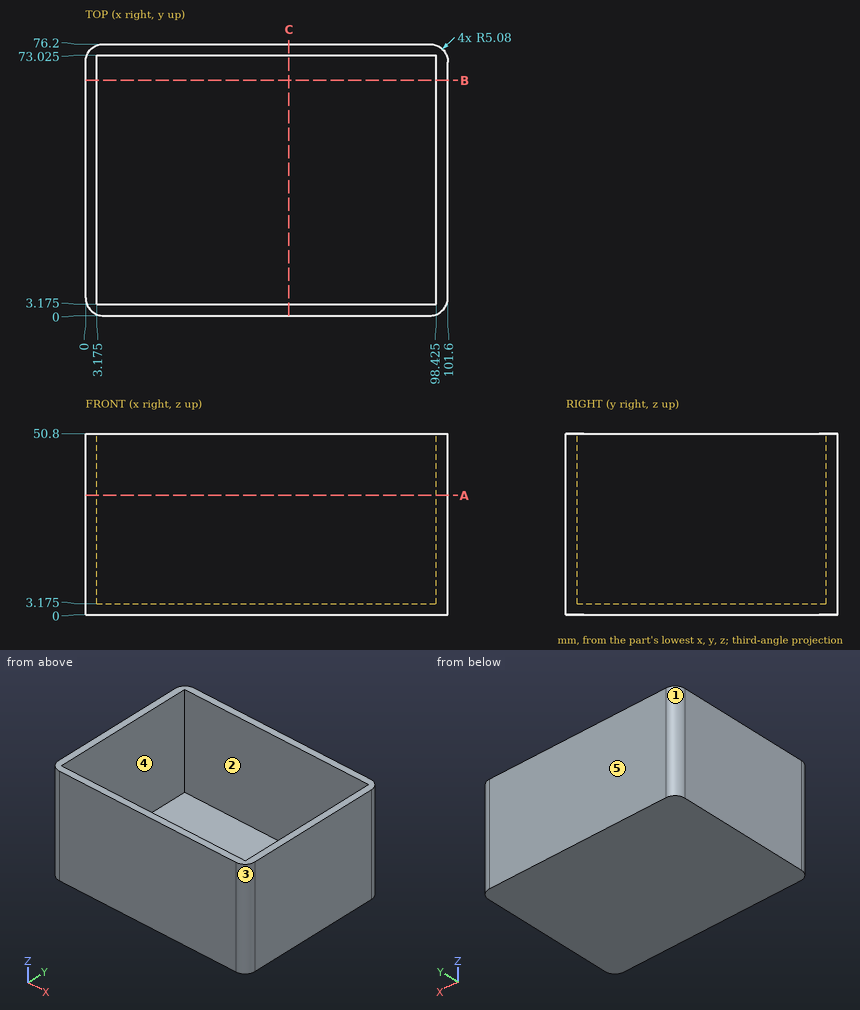
Verification items for this drawing (mm, ordinates from the low corner). A direction names the side the tool comes from. Coordinates: 2 decimals unless noted, no trailing zeros. Order: outer loops, then holes, each group sorted by start corner. A loop starts at its lowest first (then second) coordinate and runs counter-clockwise, first axis right, second up. Notation, with made-up numbers: M -7.75,11 L 18.25,11 A20 ccw 18.25,16 Z; hole C 37.25,26 d3. An arc over 180 degrees is marked long. One line per item, written item: value. Start each with the question number.
Item 1: Sectioned sample at C-C on x = 57. Record the cut outline in (y, z) (3 decimals), then the cut area to 3 significant figures.
Item 2: Access from +Z, -Z, +X, -X, +Y, -Y to the whole of each face (thin tool, end or side, straight path). Record for the marked faces 4 and 5.
Item 3: Sectioned sample at B-B on y = 66. Record the cut outline in (x, z) (3 decimals), then the cut area to 3 significant figures.
Item 4: Mould release check, pull along X, two halves, no side actions. Record for the marked faces 1, 2 and 3: pulls with the +X half, pulls with the -X half, needs draft (parallel to the pull), parting line crosses it, or undercut.
Item 5: Sectioned sample at A-A on z = 33.5. Record the cut outline in (x, y) (3 decimals).
Item 6: Depth check by flat-ended pin: P1, Ø24, axis at y = 54, z = 37.5, coming from the -X side; P2, Ø1.5, axis at x = 48.5, y = 33.5, coming from the +Z side (3 decimals). Enter the tip coordinate at first touch or a pass-through.
Item 7: Thickness scan on probe 1 along Y at (x, z) = (44.5, 18) (3 decimals); probe 2 along X at (y, z) = (54.5, 25.5) (3 decimals); probe 3 along Z at (x, y) = (24, 48) (3 decimals). Record the ranges inside material, lowest first.
Calculated:
1. outline: M 0,0 L 76.2,0 L 76.2,50.8 L 73.025,50.8 L 73.025,3.175 L 3.175,3.175 L 3.175,50.8 L 0,50.8 Z
1. area: 544 mm^2
2. face 4: +Z
2. face 5: +Z, -Z, +X, -X, +Y
3. outline: M 0,0 L 101.6,0 L 101.6,50.8 L 98.425,50.8 L 98.425,3.175 L 3.175,3.175 L 3.175,50.8 L 0,50.8 Z
3. area: 625 mm^2
4. face 1: pulls with the -X half
4. face 2: undercut
4. face 3: pulls with the +X half
5. outline: M 0,5.08 A5.08 ccw 5.08,0 L 96.52,0 A5.08 ccw 101.6,5.08 L 101.6,71.12 A5.08 ccw 96.52,76.2 L 5.08,76.2 A5.08 ccw 0,71.12 Z; hole M 3.175,3.175 L 98.425,3.175 L 98.425,73.025 L 3.175,73.025 Z
6. P1: x = 0
6. P2: z = 3.175
7. probe 1: 0 to 3.175, 73.025 to 76.2
7. probe 2: 0 to 3.175, 98.425 to 101.6
7. probe 3: 0 to 3.175
